Input: part model. Units: mm. Frame: model coordinates. Face numbers are marked on the shaded views. A direction names the side the tool comes from. Coordinates: 2 decimals unless noted, no trailing zeros. Write each loop counter-clockwise with the first axis right and the second up, starting at its lowest first coordinate (ties: lowest second). Pieces come first, ordered by that corner, then holes. Notation, with made-up numbers: (-34, 68.5) - (1, 68.5) arc R23 cw to (1, 97.5) - close; hole circle Ø6 at (41, 84). An arc over 180 degrees is marked (long way). One line per question, with ' | ' between items. Start each with the question number.
1) Line query: line 1 (Z direction, x = -2.5, y = 14.5); line 2 (Z direction, x = -6, y = 1.1). Output: solid intervals per line, ascending.
2) Section query D-D on x = -6. Return loops of the section in (y, z).
3) Section query B-B on x = -2.5. Return loops of the section in (y, z), and give its area (3 significant figures).
4) Reachability of the marked faces 1 and 2 from +Z, -Z, +X, -X, +Y, -Y: full face, straight path, thin tool, end or side. Return the list, or none.
5) First-contact query: P1, Ø1.3, axis at x = -8, y = 5.5, coming from the -Z side; P2, Ø3, axis at x = -6, z = -6, coming from the -Y side; P3, Ø1.5, axis at x = -6.5, y = 33, coming from the +Z side. Flat tips, straight axial feed; report the tip coordinate or a pass-through.
6) Section query A-A on y = 5. Return loops of the section in (x, z).
7) Section query C-C on z = -1.75. Return loops of the section in (x, y).
8) Draft query along Z for the marked faces 3, 4, 5 and 6. Return one class per face: released by +Z, released by -Z, zero draft, split by the parting line, or undercut.
Autodesk Inventor part; units mm, degrees
ref_plane "Work Plane1" through (0, 3, 0) normal (0, -1, 0) x (1, 0, 0)
ref_plane "YZ Plane" through (0, 0, 0) normal (1, 0, 0) x (0, 1, 0)
ref_plane "XZ Plane" through (0, 0, 0) normal (0, 1, 0) x (-1, 0, 0)
sketch "Sketch1" plane through (0, 0, 0) normal (0, 1, 0) x (-1, 0, 0)
  line L0 (0, -8.85) -> (0, -7.5)
  line L1 (0, -4.5) -> (0, -3.15)
  line L2 (3, -6) -> (3, -7.5)
  line L3 (3, -7.5) -> (0, -7.5)
  line L4 (0, -4.5) -> (3, -4.5)
  line L5 (3, -4.5) -> (3, -6)
  line L6 (4.5, -12) -> (4.5, -9)
  line L7 (4.5, -9) -> (6, -9)
  line L8 (6, -9) -> (7.5, -9)
  line L9 (7.5, -9) -> (7.5, -12)
  line L10 (12, -7.5) -> (9, -7.5)
  line L11 (9, -7.5) -> (9, -6)
  line L12 (9, -6) -> (9, -4.5)
  line L13 (9, -4.5) -> (12, -4.5)
  line L14 (7.5, 0) -> (7.5, -3)
  line L15 (7.5, -3) -> (6, -3)
  line L16 (6, -3) -> (4.5, -3)
  line L17 (4.5, -3) -> (4.5, 0)
  line L18 (12, 0) -> (12, -4.5)
  line L19 (12, -7.5) -> (12, -12)
  line L20 (12, -12) -> (7.5, -12)
  line L21 (4.5, -12) -> (0, -12)
  line L22 (0, 0) -> (4.5, 0)
  line L23 (7.5, 0) -> (12, 0)
  line L24 (0, -12) -> (0, -7.5)
  line L25 (0, -4.5) -> (0, 0)
  point P0 (6, -6)
  dimension "d10" = 360
  dimension "d1" = 12
extrude "Extrusion1" add sketch "Sketch1" along normal blind 50
ref_plane "Work Plane1" through (0, 3, 0) normal (0, -1, 0) x (1, 0, 0)
sketch "Sketch6" plane through (0, 3, 0) normal (0, -1, 0) x (1, 0, 0)
  line L0 (-8.6812, -4.452) -> (-7.3406, -3.678)
  line L1 (-7.3406, -3.678) -> (-6.1663, -3)
  line L2 (-6.1663, -3) -> (-5.8337, -3)
  line L3 (-5.8337, -3) -> (-4.6594, -3.678)
  line L4 (-4.6594, -3.678) -> (-3.3187, -4.452)
  line L5 (-3.3187, -4.452) -> (-3.3188, -6)
  line L6 (-3.3188, -6) -> (-3.3188, -12)
  line L7 (-3.3188, -12) -> (-4.5, -12)
  line L8 (-4.5, -12) -> (-4.5, -9)
  line L9 (-4.5, -9) -> (-7.5, -9)
  line L10 (-7.5, -9) -> (-7.5, -12)
  line L11 (-7.5, -12) -> (-8.6812, -12)
  line L12 (-8.6812, -12) -> (-8.6812, -6)
  line L13 (-8.6812, -6) -> (-8.6812, -4.452)
  point P0 (0, 0)
extrude "Extrusion2" cut sketch "Sketch6" against normal blind 4
sketch "Sketch7" plane through (0, 0, 0) normal (0, -1, 0) x (1, 0, 0)
  line L0 (0, 0) -> (0, -4.5)
  line L1 (-4.5, 0) -> (0, 0)
  line L2 (-4.5, -3) -> (-4.5, 0)
  line L3 (-7.5, -3) -> (-4.5, -3)
  line L4 (-7.5, 0) -> (-7.5, -3)
  line L5 (-12, 0) -> (-7.5, 0)
  line L6 (-12, -4.5) -> (-12, 0)
  line L7 (-9, -4.5) -> (-12, -4.5)
  line L8 (-9, -7.5) -> (-9, -4.5)
  line L9 (-12, -7.5) -> (-9, -7.5)
  line L10 (-12, -12) -> (-12, -7.5)
  line L11 (-7.5, -12) -> (-12, -12)
  line L12 (-7.5, -9) -> (-7.5, -12)
  line L13 (-4.5, -9) -> (-7.5, -9)
  line L14 (-4.5, -12) -> (-4.5, -9)
  line L15 (0, -12) -> (-4.5, -12)
  line L16 (0, -7.5) -> (0, -12)
  line L17 (-3, -7.5) -> (0, -7.5)
  line L18 (-3, -4.5) -> (-3, -7.5)
  line L19 (0, -4.5) -> (-3, -4.5)
  circle A0 centre (-6, -6) radius 1.6
  dimension "d26" = 3.2
extrude "Extrusion3" cut sketch "Sketch7" against normal blind 25.4 contours A0
sketch "Sketch8" plane through (-7.5, 0, -12) normal (0, 0, -1) x (-1, 0, 0)
  line L0 (-3, 7) -> (0, 7)
  line L1 (-3, 50) -> (0, 50)
  line L2 (-1.6663, 3) -> (-4.1813, 3)
  line L3 (-1.6663, 7) -> (-4.1813, 7)
  line L4 (-4.1813, 3) -> (-4.1813, 7)
  line L5 (0, 3) -> (-3, 3)
  line L6 (-3, 0) -> (0, 0)
  line L7 (1.1812, 3) -> (-0.1594, 3)
  line L8 (1.1812, 3) -> (1.1812, 7)
  line L9 (1.1812, 7) -> (-0.1594, 7)
  point P0 (-7.5, 0)
extrude "Extrusion4" cut sketch "Sketch8" against normal up to surface (9 mm away)
properties part number "Maze Wall Post"
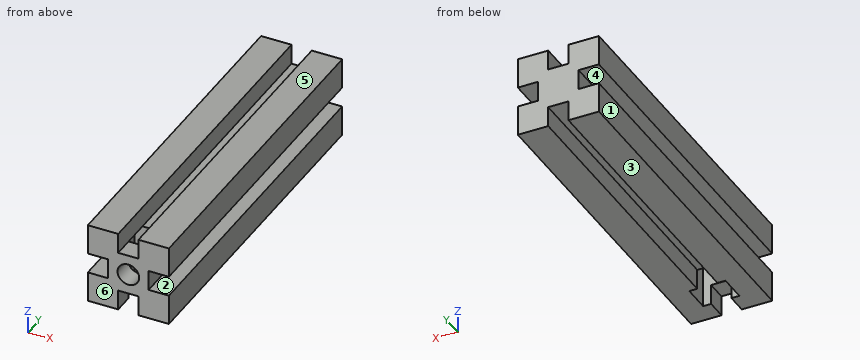
Answer key:
1) line 1: -12 to -7.5, -4.5 to 0 | line 2: -9 to -7.6, -4.4 to -3
2) outline: (0, -9) - (3, -9) - (3, -7.6) - (0, -7.6) - close; (0, -4.4) - (3, -4.4) - (3, -3) - (0, -3) - close; (7, -9) - (50, -9) - (50, -3) - (7, -3) - (7, -4.4) - (25.4, -4.4) - (25.4, -7.6) - (7, -7.6) - close
3) outline: (0, -12) - (50, -12) - (50, -7.5) - (0, -7.5) - close; (0, -4.5) - (50, -4.5) - (50, 0) - (0, 0) - close | area: 450 mm²
4) face 1: +Z, -Z, -X, +Y, -Y | face 2: +X, +Y, -Y
5) P1: z = -3 | P2: y = 25.4 | P3: z = -3
6) outline: (-12, -12) - (-8.68, -12) - (-8.68, -3) - (-7.5, -3) - (-7.5, 0) - (-12, 0) - (-12, -4.5) - (-9, -4.5) - (-9, -7.5) - (-12, -7.5) - close; (-4.5, -3) - (-3.32, -3) - (-3.32, -12) - (0, -12) - (0, -7.5) - (-3, -7.5) - (-3, -4.5) - (0, -4.5) - (0, 0) - (-4.5, 0) - close
7) outline: (-12, 0) - (-7.5, 0) - (-7.5, 50) - (-12, 50) - close; (-4.5, 0) - (0, 0) - (0, 50) - (-4.5, 50) - close
8) face 3: released by -Z | face 4: undercut | face 5: released by +Z | face 6: zero draft
